For this review, take the finished solid that the model builds, in its own axes (mm). A direction names the side the tool comes from. Round coordinates to 2 decimals unless told otherwise and drop trailing zeros. Order: outer loops, then holes, each group sorted by start corner. A loop starts at its lowest first (then second) coordinate and runs counter-clockwise, first axis right, second up. Notation, with made-up numbers: M 35.5,56.5 L 46.5,56.5 A25 cw 46.5,88.5 Z; hole C 8,27 d9. An arc over 180 degrees is marked long. Put each result on its own line as item: value.
Autodesk Inventor part; units mm, degrees
ref_plane "YZ Plane" through (0, 0, 0) normal (1, 0, 0) x (0, 1, 0)
ref_plane "XZ Plane" through (0, 0, 0) normal (0, 1, 0) x (-1, 0, 0)
ref_plane "XY Plane" through (0, 0, 0) normal (0, 0, 1) x (1, 0, 0)
sketch "Sketch1" plane through (0, 0, 0) normal (0, 0, 1) x (1, 0, 0)
  circle A0 centre (0, 0) radius 5.588
  circle A1 centre (0, 0) radius 4.318
  circle A2 centre (0, 0) radius 14.478
  circle A3 centre (0, 0) radius 15.748
  dimension "d0" = 1.27
  dimension "d1" = 11.176
  dimension "d2" = 1.27
  dimension "d3" = 8.89
extrude "Extrusion1" add sketch "Sketch1" along normal blind 14.478
sketch "Sketch3" plane through (0, 0, 14.478) normal (0, 0, 1) x (1, 0, 0)
  point P0 (0, 0)
extrude "Extrusion2" add sketch "Sketch1" along normal mid plane 1.27 contours A0 | A2
sketch "Sketch4" plane through (0, 0, -0.635) normal (0, 0, -1) x (-1, 0, 0)
  arc A0 (-6.1954, 13.0855) -> (6.1954, 13.0855) centre (0, 14.478) ccw
  arc A1 (6.1954, 13.0855) -> (-6.1954, 13.0855) centre (0, 0) ccw
  arc A2 (-14.3595, -1.8486) -> (-10.5305, 9.9358) centre (-13.7694, 4.4739) ccw
  arc A3 (-10.5305, 9.9358) -> (-14.3595, -1.8486) centre (0, 0) ccw
  arc A4 (-2.6792, -14.2279) -> (-12.7036, -6.9448) centre (-8.51, -11.7129) ccw
  arc A5 (-12.7036, -6.9448) -> (-2.6792, -14.2279) centre (0, 0) ccw
  arc A6 (12.7036, -6.9448) -> (2.6792, -14.2279) centre (8.51, -11.7129) ccw
  arc A7 (2.6792, -14.2279) -> (12.7036, -6.9448) centre (0, 0) ccw
  arc A8 (10.5305, 9.9358) -> (14.3595, -1.8486) centre (13.7694, 4.4739) ccw
  arc A9 (14.3595, -1.8486) -> (10.5305, 9.9358) centre (0, 0) ccw
  point P0 (0, 0)
  dimension "d8" = 12.7
  dimension "d11" = 360
extrude "Extrusion3" cut sketch "Sketch4" against normal blind 2.54
properties part number "WheelDE" material "PMMA Plastic"
(1) Add section A-A on z = 2.5. Give the boundary of the cut face in (x, y), then the cut area to 3 significant figures.
A:
outline: C 0,0 d31.5; C 0,0 d11.18; hole C 0,0 d28.96; hole C 0,0 d8.64
area: 160 mm2
(2) Insertion check: pin 1 Ø3 at (x, y) = (9.5, 12.5) entering from -Z (3 decimals); pin 2 Ø6 at (y, z) = (7, 12.5) entering from +X; pin 3 Ø1.5 at (x, z) = (10.5, 6.5) entering from +Y; pin 4 Ø6 at (x, z) = (10.5, 10) entering from -Y. Each pin has a flat end and moves straight along its axis. Give the tip position at first contact, or say it passes through.
A:
pin 1: stops at z = -0.635
pin 2: stops at x = 15.23
pin 3: stops at y = 12.37
pin 4: stops at y = -13.85
(3) Add section C-C on y = -3.5. Give the boundary of the cut face in (x, z) (3 decimals).
A:
outline: M -15.354,0 L -14.049,0 L -14.049,-0.635 L -2.529,-0.635 L -2.529,14.478 L -4.356,14.478 L -4.356,0.635 L -14.049,0.635 L -14.049,14.478 L -15.354,14.478 Z; M 2.529,-0.635 L 14.049,-0.635 L 14.049,0 L 15.354,0 L 15.354,14.478 L 14.049,14.478 L 14.049,0.635 L 4.356,0.635 L 4.356,14.478 L 2.529,14.478 Z
(4) For faces 1 (the face through (-8.479, 11.735, -0.313)), 2 (the face through (8.54, 11.69, -0.31)), 3 (the face through (5.3, 2.4, 0.635)), 4 (the face through (-0.09, 14.478, 0.313)), list the 3-axis set-ups (+Z, -Z, +X, -X, +Y, -Y) from which the entire face can be reached by the end or side of a thin tool; tool diameter is ignored.
A:
face 1: -Z, -X, +Y
face 2: -Z, +X, +Y
face 3: +Z
face 4: +Z, -Z
(5) Add section B-B on y = 0. Give the boundary of the cut face in (x, z) (3 decimals), then the cut area to 3 significant figures.
A:
outline: M -15.748,0 L -14.478,0 L -14.478,14.478 L -15.748,14.478 Z; M -9.263,-0.635 L -4.318,-0.635 L -4.318,14.478 L -5.588,14.478 L -5.588,0.635 L -9.263,0.635 Z; M 4.318,-0.635 L 9.263,-0.635 L 9.263,0.635 L 5.588,0.635 L 5.588,14.478 L 4.318,14.478 Z; M 14.478,0 L 15.748,0 L 15.748,14.478 L 14.478,14.478 Z
area: 84.5 mm2
(6) Add section D-D on x = 0. Give the boundary of the cut face in (y, z) (3 decimals).
A:
outline: M -15.748,0 L -14.478,0 L -14.478,-0.635 L -4.318,-0.635 L -4.318,14.478 L -5.588,14.478 L -5.588,0.635 L -14.478,0.635 L -14.478,14.478 L -15.748,14.478 Z; M 4.318,-0.635 L 8.128,-0.635 L 8.128,0.635 L 5.588,0.635 L 5.588,14.478 L 4.318,14.478 Z; M 14.478,0 L 15.748,0 L 15.748,14.478 L 14.478,14.478 Z
(7) To check wall thickness, follow L1, parallel to Y at x = 0, z = 4.5; L2, parallel to X at y = 5, z = 8.25; L3, parallel to Y at x = 1.5, z = 8.75. State the ranges of each line that lie inside material, in increasing order.
A:
L1: y = -15.75 to -14.48, -5.59 to -4.32, 4.32 to 5.59, 14.48 to 15.75
L2: x = -14.93 to -13.59, -2.5 to 2.5, 13.59 to 14.93
L3: y = -15.68 to -14.4, -5.38 to -4.05, 4.05 to 5.38, 14.4 to 15.68
